The model under review builds one solid part; all positions refer to its coordinate system, in mm. A direction names the side the tool comes from. Coordinates: 2 decimals unless noted, no trailing zeros. Order: outer loops, then holes, each group sorted by start corner. A loop starts at its lowest first (then second) coordinate and runs counter-clockwise, first axis right, second up. Notation, with made-up numbers: (0.5, 54.5) - (24.5, 54.5) arc R19 ccw to (24.5, 58.5) - close; hole circle Ø4 at (39, -19). An arc over 180 degrees is marked (long way). Answer in a Markdown table with one row per item.
```python
from build123d import *

# Parameters (mm, degrees)
EXTRUDE_1_DEPTH          = 6
CUT_EXTRUDE_1_DEPTH      = 18.464249197
CUT_EXTRUDE_1_DEPTH_BACK = 18.464249197
SKETCH_2_R               = 1.6
SKETCH_3_R               = 2.8
CUT_EXTRUDE_2_DEPTH      = 17.733200638
CUT_EXTRUDE_3_DEPTH      = 17.031219648


with BuildPart() as part:
    # 草图1 → 凸台-拉伸1 (new body)
    with BuildSketch(Plane.XY):
        with BuildLine():
            Line((-5, 7.141428429), (-5, 10))
            Line((-5, 10), (-0.8, 10))
            Line((-0.8, 10), (-0.8, 5.363068152))
            ThreePointArc((-0.8, 5.363068152), (-1.089555662, 4.326545038), (-1.874380165, 3.59015306))
            ThreePointArc((-1.874380165, 3.59015306), (0, -4.05), (1.874380165, 3.59015306))
            ThreePointArc((1.874380165, 3.59015306), (1.089555662, 4.326545038), (0.8, 5.363068152))
            Line((0.8, 5.363068152), (0.8, 10))
            Line((0.8, 10), (5, 10))
            Line((5, 10), (5, 7.141428429))
            ThreePointArc((5, 7.141428429), (5.156091109, 6.366831759), (5.6, 5.713142743))
            ThreePointArc((5.6, 5.713142743), (0, -8), (-5.6, 5.713142743))
            ThreePointArc((-5.6, 5.713142743), (-5.156091109, 6.366831759), (-5, 7.141428429))
        make_face()
    extrude(amount=EXTRUDE_1_DEPTH)

    # 草图2 → 切除-拉伸1 (cut, two sides: drawn at the far end of the back side and taken through both)
    with BuildSketch(Plane.ZY.offset(5).offset(-CUT_EXTRUDE_1_DEPTH_BACK)):
        with Locations(Location((3, 7, 0), (0, 0, 5.071150936))):
            Circle(SKETCH_2_R)
    extrude(amount=CUT_EXTRUDE_1_DEPTH + CUT_EXTRUDE_1_DEPTH_BACK, mode=Mode.SUBTRACT)

    # 草图3 → 切除-拉伸2 (cut, through all)
    with BuildSketch(Plane.ZY.offset(4)):
        with Locations(Location((3, 7, 0), (0, 0, 177.10474942))):
            Circle(SKETCH_3_R)
    extrude(amount=CUT_EXTRUDE_2_DEPTH, mode=Mode.SUBTRACT)

    # 草图4 → 切除-拉伸3 (cut, through all)
    with BuildSketch(Plane(origin=(3, 0, 0), x_dir=(0, 0, -1), z_dir=(1, 0, 0))):
        Polygon((0.233161507, 7), (-1.383419246, 9.8), (-4.616580754, 9.8), (-6.233161507, 7), (-4.616580754, 4.2), (-1.383419246, 4.2), align=None)
    extrude(amount=CUT_EXTRUDE_3_DEPTH, mode=Mode.SUBTRACT)


solid = part.part
```
Item 1: We need section C-C, the plane z = 2. Write out the cut boundary in (x, y), then the cut area to 3 significant figures.
Check values:
| item | result |
|---|---|
| outline | (-6.69, 4.38) arc R8 ccw (long way) to (6.81, 4.2) - (3, 4.2) - (3, 5.75) - (0.8, 5.75) - (0.8, 5.36) arc R2 ccw to (1.87, 3.59) arc R4.05 cw (long way) to (-1.87, 3.59) arc R2 ccw to (-0.8, 5.36) - (-0.8, 5.75) - (-4, 5.75) - (-4, 4.38) - close; (-5, 9.62) - (-4, 9.62) - (-4, 8.25) - (-0.8, 8.25) - (-0.8, 10) - (-5, 10) - close; (0.8, 8.25) - (3, 8.25) - (3, 9.8) - (5, 9.8) - (5, 10) - (0.8, 10) - close |
| area | 131 mm^2 |
Item 2: Clearance check with flat-ended pins moving along their axes: pin 1 Ø2.5 at (y, z) = (7.5, 3) entering from +X; pin 2 Ø3 at (y, z) = (8, 4) entering from -X; pin 3 Ø3 at (y, z) = (-5, 1.5) entering from +X. State where each tip first meets the part, or that it passes through.
Check values:
| item | result |
|---|---|
| pin 1 | x = 3 |
| pin 2 | x = -5 |
| pin 3 | x = 7.19 |
Item 3: To check wall thickness, follow line 1 (X direction, y = 0, z = 1.9); line 2 (X direction, y = 6.5, z = 5.5); line 3 (Z direction, x = -2.4, y = 7). State the ranges of each line that lie inside material, in increasing order. Write a range as from..to.
Check values:
| item | result |
|---|---|
| line 1 | -8..-4.05, 4.05..8 |
| line 2 | -4..-0.8, 0.8..3 |
| line 3 | 0..1.4, 4.6..6 |
Item 4: We need section D-D, the plane x = 3.25. Write out the cut boundary in (y, z), then the cut area to 3 significant figures.
Check values:
| item | result |
|---|---|
| outline | (-7.31, 0) - (-2.42, 0) - (-2.42, 6) - (-7.31, 6) - close; (2.42, 0) - (6.6, 0) - (4.2, 1.38) - (4.2, 4.62) - (6.6, 6) - (2.42, 6) - close; (7.4, 0) - (10, 0) - (10, 6) - (7.4, 6) - (9.8, 4.62) - (9.8, 1.38) - close |
| area | 47.9 mm^2 |
Item 5: We need section A-A, the plane x = -1. Write out the cut boundary in (y, z).
Check values:
| item | result |
|---|---|
| outline | (-7.94, 0) - (-3.92, 0) - (-3.92, 6) - (-7.94, 6) - close; (4.49, 0) - (10, 0) - (10, 6) - (4.49, 6) - close; hole circle Ø3.2 at (7, 3) |
Item 6: Tool access review of faces 5 (the face through (-3, 3, 0)), 6 (the face through (3.986, 8.585, 0.682)), 7 (the face through (1.1, 4.31, 2.96)), 8 (the face through (0.8, 9, 3)), 9 (the face through (-4, 7, 1)): name each direction out of +Z, -Z, +X, -X, +Y, -Y from which nothing blocks a thin tool from reaching the whole face with its end or side.
Check values:
| item | result |
|---|---|
| face 5 | -Z, +X, -X, +Y, -Y |
| face 6 | +X |
| face 7 | +Z, -Z |
| face 8 | +Z, -Z, +Y |
| face 9 | -X |
Item 7: We need section B-B, the plane y = 0. Write out the cut boundary in (x, z), then the cut area to 3 significant figures.
Check values:
| item | result |
|---|---|
| outline | (-8, 0) - (-4.05, 0) - (-4.05, 6) - (-8, 6) - close; (4.05, 0) - (8, 0) - (8, 6) - (4.05, 6) - close |
| area | 47.4 mm^2 |
Item 8: Mouldability with a two-part tool opening along X and no side actions: class faces 1 (the face through (1.915, 5.414, 2.793)), 2 (the face through (-5, 9.73, 1.87)), 3 (the face through (-0.151, -4.047, 2.958)), 4 (the face through (3, 8.3, 4.4)) as +X half, -X half, draft (parallel to the pull), parting line (faces both ways), or undercut.
Check values:
| item | result |
|---|---|
| face 1 | draft |
| face 2 | -X half |
| face 3 | undercut |
| face 4 | +X half |
